```python
from build123d import *

# Parameters (mm, degrees)
SKETCH1_W           = 80
SKETCH1_H           = 50
BOSS_EXTRUDE1_DEPTH = 1.5
SKETCH6_W           = 1.5
SKETCH6_H           = 20
BOSS_EXTRUDE4_DEPTH = 8
SKETCH8_W           = 8
SKETCH8_H           = 1.5
BOSS_EXTRUDE5_DEPTH = 35
SKETCH9_R           = 0.815
CUT_EXTRUDE2_DEPTH  = 80.368828479


with BuildPart() as part:
    # Sketch1 → Boss-Extrude1 (new body)
    with BuildSketch(Plane.XY):
        with Locations((13.251028807, -5.452674897)):
            Rectangle(SKETCH1_W, SKETCH1_H)
    extrude(amount=BOSS_EXTRUDE1_DEPTH)

    # Sketch6 → Boss-Extrude4 (add)
    with BuildSketch(Plane(origin=(53.251028807, 0, 0), x_dir=(0, 0, -1), z_dir=(1, 0, 0))):
        with Locations((-0.75, -5.452674897)):
            Rectangle(SKETCH6_W, SKETCH6_H)
    extrude(amount=BOSS_EXTRUDE4_DEPTH)

    # Sketch8 → Boss-Extrude5 (add)
    with BuildSketch(Plane.XZ.offset(15.452674897)):
        with Locations((57.251028807, 0.75)):
            Rectangle(SKETCH8_W, SKETCH8_H)
    extrude(amount=BOSS_EXTRUDE5_DEPTH)

    # Sketch9 → Cut-Extrude2 (cut, through all)
    with BuildSketch(Plane(origin=(0, 0, 0), x_dir=(-1, 0, 0), z_dir=(0, 0, -1))):
        with Locations(Location((-57.251028807, -35.452674897, 0), (0, 0, 90))):
            Circle(SKETCH9_R)
    extrude(amount=-CUT_EXTRUDE2_DEPTH, mode=Mode.SUBTRACT)


solid = part.part
```
Here's how the part is built. I have some questions about the finished solid (model axes, mm). Give positions to 0.01 mm unless a question says otherwise; leave off trailing zeros. Write each loop counter-clockwise with the first axis right and the second up, starting at its lowest first coordinate (ties: lowest second). Pieces come first, ordered by that corner, then holes. Notation, with made-up numbers: (61, 33.25) -> (120, 33.25) arc R15 ccw to (120, 56.25) -> close; hole circle Ø4 at (60.25, 51). An arc over 180 degrees is marked (long way). Use one line per item in the form item = value.
1) Suppose I cut it at C-C (x = 50). Please give me the cut outline in (y, z).
Verdict:
outline = (-30.45, 0) -> (19.55, 0) -> (19.55, 1.5) -> (-30.45, 1.5) -> close
2) Suppose I cut it at A-A (z = 0.8). Please give me the cut outline in (x, y) (3 decimals).
Verdict:
outline = (-26.749, -30.453) -> (53.251, -30.453) -> (53.251, -50.453) -> (61.251, -50.453) -> (61.251, 4.547) -> (53.251, 4.547) -> (53.251, 19.547) -> (-26.749, 19.547) -> close; hole circle Ø1.63 at (57.251, -35.453)
3) If I drill on L1, parallel to Y at x = 22, z = 0.45; L2, parallel to X at y = -36, z = 0.1; L3, parallel to X at y = 6, z = 0.4, over which ranges is the centre line in solid material (lowest first)? Write a range as [from, to].
Verdict:
L1 = [-30.45, 19.55]
L2 = [53.25, 56.65], [57.85, 61.25]
L3 = [-26.75, 53.25]
4) Suppose I cut it at B-B (y = -41.5). Please give me the cut outline in (x, z), and give its area (3 significant figures).
Verdict:
outline = (53.25, 0) -> (61.25, 0) -> (61.25, 1.5) -> (53.25, 1.5) -> close
area = 12.0 mm2
